For this review, take the finished solid that the model builds, in its own axes (mm). A direction names the side the tool comes from. Coordinates: 2 decimals unless noted, no trailing zeros. Write each loop counter-clockwise with the first axis right and the second up, starting at its lowest first coordinate (ties: lowest second). Pieces come first, ordered by that corner, then holes.
```python
from build123d import *

# Parameters (mm, degrees)
SKETCH1_W           = 16
SKETCH1_H           = 30
BOSS_EXTRUDE1_DEPTH = 6.5
SKETCH3_R           = 1.09
CUT_EXTRUDE1_DEPTH  = 7.5
FILLET1_R           = 2
SKETCH5_W           = 10
SKETCH5_H           = 7.5
BOSS_EXTRUDE2_DEPTH = 6.5
FILLET2_R           = 2
FILLET3_R           = 2
FILLET4_R           = 2
SKETCH4_R           = 1.13
CUT_EXTRUDE2_DEPTH  = 31


with BuildPart() as part:
    # Sketch1 → Boss-Extrude1 (new body)
    with BuildSketch(Plane.XY):
        with Locations((8, 15)):
            Rectangle(SKETCH1_W, SKETCH1_H)
    extrude(amount=BOSS_EXTRUDE1_DEPTH)

    # Sketch3 → Cut-Extrude1 (cut, through all)
    with BuildSketch(Plane(origin=(0, 0, 0), x_dir=(-1, 0, 0), z_dir=(0, 0, -1))):
        with Locations((-13.5, 6.87)):
            Circle(SKETCH3_R)
        with Locations((-2.5, 6.87)):
            Circle(SKETCH3_R)
        with Locations((-2.5, 24.87)):
            Circle(SKETCH3_R)
        with Locations((-13.5, 24.87)):
            Circle(SKETCH3_R)
    extrude(amount=-CUT_EXTRUDE1_DEPTH, mode=Mode.SUBTRACT)

    # Fillet1
    fillet1_edges = [part.edges().sort_by_distance(p)[0] for p in [
        (0, 30, 3.25),
        (16, 30, 3.25),
    ]]
    fillet(fillet1_edges, radius=FILLET1_R)

    # Sketch5 → Boss-Extrude2 (add)
    with BuildSketch(Plane.XY.offset(6.5)):
        with Locations((-5, 3.75)):
            Rectangle(SKETCH5_W, SKETCH5_H)
        with Locations((21, 3.75)):
            Rectangle(SKETCH5_W, SKETCH5_H)
    extrude(amount=-BOSS_EXTRUDE2_DEPTH)

    # Fillet2
    fillet2_edges = [part.edges().sort_by_distance(p)[0] for p in [
        (0, 7.5, 3.25),
        (16, 7.5, 3.25),
    ]]
    fillet(fillet2_edges, radius=FILLET2_R)

    # Fillet3
    fillet3_edges = [part.edges().sort_by_distance(p)[0] for p in [
        (26, 7.5, 3.25),
    ]]
    fillet(fillet3_edges, radius=FILLET3_R)

    # Fillet4
    fillet4_edges = [part.edges().sort_by_distance(p)[0] for p in [
        (-10, 7.5, 3.25),
    ]]
    fillet(fillet4_edges, radius=FILLET4_R)

    # Sketch4 → Cut-Extrude2 (cut, through all)
    with BuildSketch(Plane.XZ):
        with Locations((20.5, 3.25)):
            Circle(SKETCH4_R)
        with Locations((-4.5, 3.25)):
            Circle(SKETCH4_R)
    extrude(amount=-CUT_EXTRUDE2_DEPTH, mode=Mode.SUBTRACT)


solid = part.part
```
Q1. Tool access review of faces 1 (the cylindrical face through (15.4, 29.43, 3.3)), 2 (the flat face through (0, 19, 3)): name each direction out of +Z, -Z, +X, -X, +Y, -Y from which nothing blocks a thin tool from reaching the whole face with its end or side.
Ans:
face 1: +Z, -Z, +X, +Y
face 2: +Z, -Z, -X, +Y
Q2. Clearance check with flat-ended pins moving along their axes: pin 1 Ø2.5 at (x, y) = (2.5, 24.87) entering from +Z; pin 2 Ø1.5 at (y, z) = (13.5, 3) entering from +X; pin 3 Ø1.8 at (x, z) = (-4.5, 2.5) entering from +Y. State where each tip first meets the part, or that it passes through.
Ans:
pin 1: stops at z = 6.5
pin 2: stops at x = 16
pin 3: stops at y = 7.5
Q3. Add section D-D (y = 6.87). State the section outline as (x, z) points, then the cut area to 3 significant figures.
Ans:
outline: (-9.46, 0) - (1.41, 0) - (1.41, 6.5) - (-9.46, 6.5) - close; (3.59, 0) - (12.41, 0) - (12.41, 6.5) - (3.59, 6.5) - close; (14.59, 0) - (25.46, 0) - (25.46, 6.5) - (14.59, 6.5) - close; hole circle Ø2.26 at (-4.5, 3.25); hole circle Ø2.26 at (20.5, 3.25)
area: 191 mm2
Q4. Add section A-A (y = 24.87). State the section outline as (x, z) points, then the cut area to 3 significant figures.
Ans:
outline: (0, 0) - (1.41, 0) - (1.41, 6.5) - (0, 6.5) - close; (3.59, 0) - (12.41, 0) - (12.41, 6.5) - (3.59, 6.5) - close; (14.59, 0) - (16, 0) - (16, 6.5) - (14.59, 6.5) - close
area: 75.7 mm2
Q5. Draft analysis for pull direction X (two halves, no side actions). For faces 3 (the flat face through (16, 19, 3)), 4 (the cylindrical face through (-5.63, 3.7, 3.3)), 5 (the flat face through (-10, 3, 3)), state which applies: +X half, -X half, draft (parallel to the pull), parting line (faces both ways), or undercut.
Ans:
face 3: +X half
face 4: undercut
face 5: -X half
Q6. For probe 1 along Z at (x, y) = (20.5, 4.5); probe 2 along Y at (x, z) = (13.5, 4.25); probe 3 along X at (y, z) = (3, 4), list the stretches that pass through material, from the lowest coordinate up.
Ans:
probe 1: z = 0 to 2.12, 4.38 to 6.5
probe 2: y = 0 to 5.78, 7.96 to 23.78, 25.96 to 30
probe 3: x = -10 to -5.35, -3.65 to 19.65, 21.35 to 26
Q7. Add section B-B (z = 3.25). State the section outline as (x, y) points.
Ans:
outline: (-10, 0) - (-5.63, 0) - (-5.63, 7.5) - (-8, 7.5) arc R2 ccw to (-10, 5.5) - close; (-3.37, 0) - (19.37, 0) - (19.37, 7.5) - (18, 7.5) arc R2 cw to (16, 9.5) - (16, 28) arc R2 ccw to (14, 30) - (2, 30) arc R2 ccw to (0, 28) - (0, 9.5) arc R2 cw to (-2, 7.5) - (-3.37, 7.5) - close; (21.63, 0) - (26, 0) - (26, 5.5) arc R2 ccw to (24, 7.5) - (21.63, 7.5) - close; hole circle Ø2.18 at (2.5, 6.87); hole circle Ø2.18 at (2.5, 24.87); hole circle Ø2.18 at (13.5, 6.87); hole circle Ø2.18 at (13.5, 24.87)
Q8. Add section C-C (x = 13.5). State the section outline as (y, z) points, then the cut area to 3 significant figures.
Ans:
outline: (0, 0) - (5.78, 0) - (5.78, 6.5) - (0, 6.5) - close; (7.96, 0) - (23.78, 0) - (23.78, 6.5) - (7.96, 6.5) - close; (25.96, 0) - (30, 0) - (30, 6.5) - (25.96, 6.5) - close
area: 167 mm2
